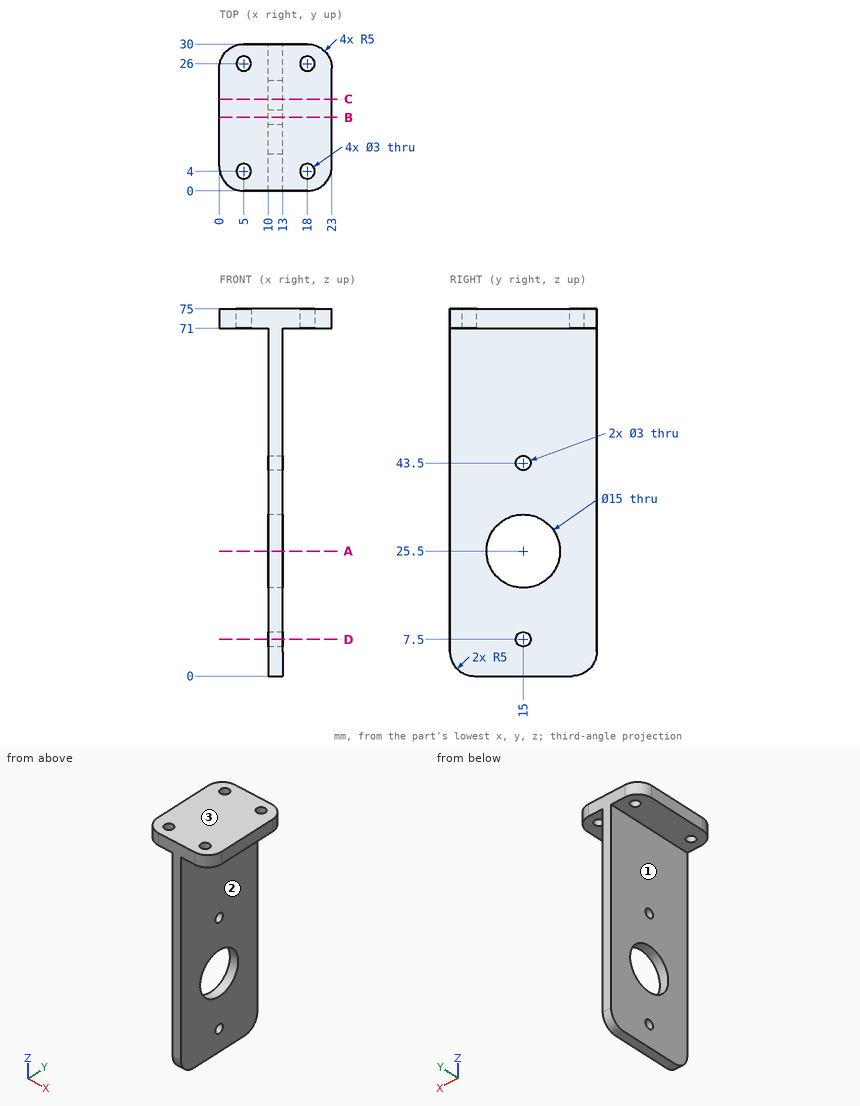
Input: dimensioned drawing with shaded views. Units: mm. Origin: part minimum x, y, z. A direction names the side the tool comes from. Round coordinates to 2 decimals unless told otherwise and drop trailing zeros. Loops run counter-clockwise (first coordinate to the right, second up) from the corner with the lowest first, then second, coordinate; pieces in that order, holes last. Notation, with made-up numbers: M 56.5,35.5 L 103.5,35.5 A22 ccw 103.5,67.5 Z; hole C -18.5,51.25 d3. An arc over 180 degrees is marked long. Answer in a Markdown table with one row per item. Add a question column.
1. Set-up query: the marked faces 1, 2 and 3. Return all of +Z, -Z, +X, -X, +Y, -Y with unobstructed straight access to the full face (end or side cutting, diameter ignored); none if empty.
2. Section D-D (z = 7.5). Output: boundary loops of the cut face in (x, y).
3. Contact query for flat-ended pins moving along their axis: pin 1 (3 mm diameter, centred on y = 14, z = 16, fed in from +X); pin 2 (3.5 mm diameter, centred on x = 18, y = 26, fed in from -Z); pin 3 (4 mm diameter, centred on y = 15, z = 43.5, fed in from -X); pin 4 (2.5 mm diameter, centred on y = 15, z = 7.5, fed in from +X). Output: stop coordinate, or through.
4. Section B-B (y = 15). Output: boundary loops of the cut face in (x, z), and give its area (3 significant figures).
5. Section A-A (z = 25.5). Output: boundary loops of the cut face in (x, y), and give its area (3 significant figures).
6. Ray query, probe 1 along Y at (x, z) = (5, 74); probe 2 along Y at (x, z) = (11, 43.5); probe 3 along Y at (x, z) = (11, 25.5). Return the intervals inside material, ascending.
7. Section C-C (y = 18.75). Output: boundary loops of the cut face in (x, z).
Values follow:
| question | item | result |
|---|---|---|
| 1 | face 1 | -Z, -X, +Y, -Y |
| 1 | face 2 | -Z, +X, +Y, -Y |
| 1 | face 3 | +Z, +X, -X, +Y, -Y |
| 2 | outline | M 10,0 L 13,0 L 13,13.5 L 10,13.5 Z; M 10,16.5 L 13,16.5 L 13,30 L 10,30 Z |
| 3 | pin 1 | x = 13 |
| 3 | pin 2 | z = 71 |
| 3 | pin 3 | x = 10 |
| 3 | pin 4 | through |
| 4 | outline | M 0,71 L 10,71 L 10,45 L 13,45 L 13,71 L 23,71 L 23,75 L 0,75 Z; M 10,0 L 13,0 L 13,6 L 10,6 Z; M 10,9 L 13,9 L 13,18 L 10,18 Z; M 10,33 L 13,33 L 13,42 L 10,42 Z |
| 4 | area | 242 mm^2 |
| 5 | outline | M 10,0 L 13,0 L 13,7.5 L 10,7.5 Z; M 10,22.5 L 13,22.5 L 13,30 L 10,30 Z |
| 5 | area | 45.0 mm^2 |
| 6 | probe 1 | 0 to 2.5, 5.5 to 24.5, 27.5 to 30 |
| 6 | probe 2 | 0 to 13.5, 16.5 to 30 |
| 6 | probe 3 | 0 to 7.5, 22.5 to 30 |
| 7 | outline | M 0,71 L 10,71 L 10,32 L 13,32 L 13,71 L 23,71 L 23,75 L 0,75 Z; M 10,0 L 13,0 L 13,19 L 10,19 Z |
